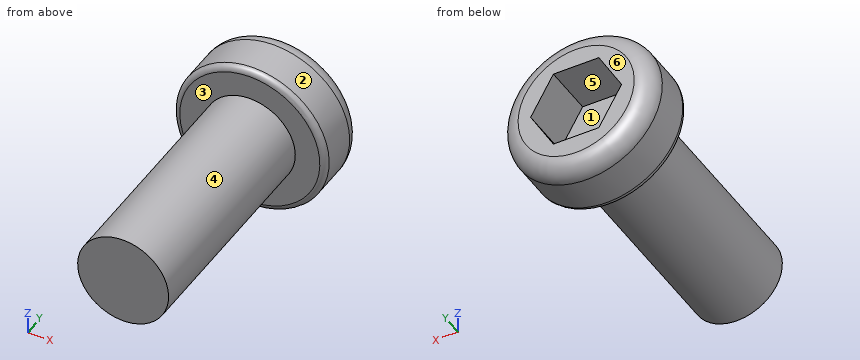
from build123d import *

# Parameters (mm, degrees)
SKETCH1_R           = 3.175
BOSS_EXTRUDE3_DEPTH = 2.5
CUT_EXTRUDE3_DEPTH  = 2.15
SKETCH8_R           = 1.9
BOSS_EXTRUDE4_DEPTH = 9.3
FILLET2_R           = 0.75
FILLET3_R           = 0.25


with BuildPart() as part:
    # Sketch1 → Boss-Extrude3 (new body)
    with BuildSketch(Plane(origin=(0, 0, 0), x_dir=(1, 0, 0), z_dir=(0, 1, 0))):
        with Locations(Location((0, 0, 0), (0, 0, 270))):
            Circle(SKETCH1_R)
    extrude(amount=BOSS_EXTRUDE3_DEPTH)

    # Sketch7 → Cut-Extrude3 (cut)
    with BuildSketch(Plane(origin=(0, 2.5, 0), x_dir=(1, 0, 0), z_dir=(0, 1, 0))):
        Polygon((0.95, 1.645448267), (-0.95, 1.645448267), (-1.9, 0), (-0.95, -1.645448267), (0.95, -1.645448267), (1.9, 0), align=None)
    extrude(amount=-CUT_EXTRUDE3_DEPTH, mode=Mode.SUBTRACT)

    # Sketch8 → Boss-Extrude4 (add)
    with BuildSketch(Plane(origin=(0, 0, 0), x_dir=(1, 0, 0), z_dir=(0, 1, 0))):
        with Locations(Location((0, 0, 0), (0, 0, 270))):
            Circle(SKETCH8_R)
    extrude(amount=-BOSS_EXTRUDE4_DEPTH)

    # Fillet2
    fillet2_edges = [part.edges().sort_by_distance(p)[0] for p in [
        (0, 2.5, -3.175),
    ]]
    fillet(fillet2_edges, radius=FILLET2_R)

    # Fillet3
    fillet3_edges = [part.edges().sort_by_distance(p)[0] for p in [
        (0, 0, -3.175),
    ]]
    fillet(fillet3_edges, radius=FILLET3_R)


solid = part.part
The model under review builds one solid part; all positions refer to its coordinate system, in mm. Face numbers are marked on the shaded views. A direction names the side the tool comes from. Coordinates: 2 decimals unless noted, no trailing zeros. Loops run counter-clockwise (first coordinate to the right, second up) from the corner with the lowest first, then second, coordinate; pieces in that order, holes last. Notation, with made-up numbers: (76, -27) -> (123, -27) arc R11 ccw to (123, -18) -> close; hole circle Ø1 at (19.25, 7.25). An arc over 180 degrees is marked (long way). Use a Markdown table: item, result. Add a question column.
1. Machinability: for the marked faces 1, 2 and 3, which of the approach directions +Z, -Z, +X, -X, +Y, -Y give a long, thin tool a straight path to every point of the face, cutting with its end or side? Answer none if there is none.
2. To check wall thickness, follow line 1 (Y direction, x = -2, z = 1); line 2 (Y direction, x = 0.75, z = 0.5); line 3 (X direction, y = -7.5, z = 0). State the ranges of each line that lie inside material, in increasing order.
3. Clearance check with flat-ended pins moving along their axes: pin 1 Ø1.6 at (x, z) = (0, 0) entering from +Y; pin 2 Ø1.5 at (y, z) = (-5, -2) entering from +X; pin 3 Ø2 at (y, z) = (-6, -2) entering from -X. State where each tip first meets the part, or that it passes through.
4. Add section B-B on y = -3. Write out the cut boundary in (x, z), plus the area to 3 significant figures.
5. Add section A-A on x = 0. Write out the cut boundary in (y, z) (3 decimals).
6. Draft analysis for pull direction X (two halves, no side actions). For the marked faces 4, 5 and 6, state which applies: pulls with the +X half, pulls with the -X half, needs draft (parallel to the pull), parting line crosses it, or undercut.
Returned:
| question | item | result |
|---|---|---|
| 1 | face 1 | +Y |
| 1 | face 2 | +Y, -Y |
| 1 | face 3 | -Y |
| 2 | line 1 | y = 0 to 2.5 |
| 2 | line 2 | y = -9.3 to 0.35 |
| 2 | line 3 | x = -1.9 to 1.9 |
| 3 | pin 1 | stops at y = 0.35 |
| 3 | pin 2 | stops at x = 1.43 |
| 3 | pin 3 | stops at x = -1.62 |
| 4 | outline | circle Ø3.8 at (0, 0) |
| 4 | area | 11.3 mm² |
| 5 | outline | (-9.3, -1.9) -> (0, -1.9) -> (0, -2.925) arc R0.25 ccw to (0.25, -3.175) -> (1.75, -3.175) arc R0.75 ccw to (2.5, -2.425) -> (2.5, -1.645) -> (0.35, -1.645) -> (0.35, 1.645) -> (2.5, 1.645) -> (2.5, 2.425) arc R0.75 ccw to (1.75, 3.175) -> (0.25, 3.175) arc R0.25 ccw to (0, 2.925) -> (0, 1.9) -> (-9.3, 1.9) -> close |
| 6 | face 4 | parting line crosses it |
| 6 | face 5 | undercut |
| 6 | face 6 | needs draft |
